Here's how the part is built. I have some questions about the finished solid (model axes, mm). Face numbers are marked on the shaded views. Round coordinates to 2 decimals unless told otherwise and drop trailing zeros. Order: outer loops, then holes, each group sorted by start corner. A loop starts at its lowest first (then second) coordinate and runs counter-clockwise, first axis right, second up. Notation, with made-up numbers: (17.5, 56) - (37.5, 56) arc R8 ccw to (37.5, 69) - close; hole circle Ø7 at (-6, -34.75). An arc over 180 degrees is marked (long way). One line per item, written item: value.
from build123d import *

# Parameters (mm, degrees)
F0_W     = 168.5284674168
F0_H     = 57.090960443
F1_DEPTH = 127
F2_R     = 6.35
F4_DEPTH = 31.75


# Not quite as in the source:
# - the program builds the solid bodies; features that only make, move or delete a surface that nothing else refers to are left out


with BuildPart() as f1:
    # F0 (on Top) → F1 (new body)
    with BuildSketch(Plane.XY):
        with Locations((20.6451192498, 11.0519304872)):
            Rectangle(F0_W, F0_H)
    extrude(amount=F1_DEPTH)

    # F2 (on Front) → F4 (join)
    with BuildSketch(Plane.XZ):
        with Locations((-52.945434434, 116.5131386886)):
            Circle(F2_R)
        with Locations((94.4893505254, 116.5369517954)):
            Circle(F2_R)
    extrude(amount=F4_DEPTH)


solid = f1.part
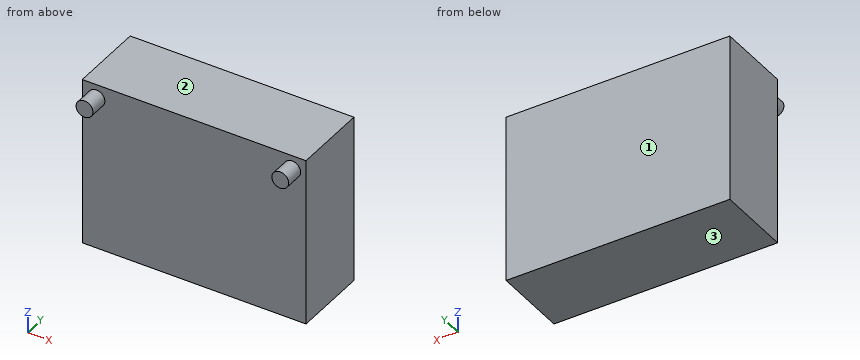
Q1. If we section it at A-A, the plane x = -51: Please give me the cut outline in (y, z), then the cut area to 3 significant figures.
Results list:
outline: (-31.75, 110.47) - (-17.49, 110.47) - (-17.49, 0) - (39.6, 0) - (39.6, 127) - (-17.49, 127) - (-17.49, 122.56) - (-31.75, 122.56) - close
area: 7,420 mm²
Q2. If we section it at B-B, the plane z = 114: Please give me the cut outline in (x, y).
Results list:
outline: (-63.62, -17.49) - (-58.78, -17.49) - (-58.78, -31.75) - (-47.11, -31.75) - (-47.11, -17.49) - (88.67, -17.49) - (88.67, -31.75) - (100.31, -31.75) - (100.31, -17.49) - (104.91, -17.49) - (104.91, 39.6) - (-63.62, 39.6) - close
Q3. If I drill on line 1 along Y through (x, z) = (-17, 59); line 2 along X through (y, z) = (-18.5, 118), over which ranges is the centre line in solid material (lowest first)?
Results list:
line 1: -17.49 to 39.6
line 2: -59.12 to -46.77, 88.31 to 100.67
Q4. We'd pull the mould along Z, two halves only. Please class the marked faces 1, 2 and 3: released by +Z, released by -Z, zero draft, split by the parting line, or undercut.
Results list:
face 1: zero draft
face 2: released by +Z
face 3: released by -Z
Q5. Will this pin go through, and if not, where does the flat tip stop? pin 1 (12 mm diameter, centred on x = 69.5, z = 78, fed in from -Y).
Results list:
pin 1: y = -17.49
Q6. If we section it at C-C, the plane x = 29: Please give me the cut outline in (y, z).
Results list:
outline: (-17.49, 0) - (39.6, 0) - (39.6, 127) - (-17.49, 127) - close
